```python
from build123d import *

# Parameters (mm, degrees)
SKETCH_1_W               = 65
SKETCH_1_H               = 25
EXTRUDE_1_DEPTH          = 20
EXTRUDE_2_DEPTH          = 65
SKETCH_3_W               = 50
SKETCH_3_H               = 20
CUT_EXTRUDE_1_DEPTH      = 15
CUT_EXTRUDE_2_DEPTH      = 50.33938589
CUT_EXTRUDE_2_DEPTH_BACK = 50.33938589
SKETCH_4_R               = 1.6
CUT_EXTRUDE_START        = -7
SKETCH_5_R               = 2.9
CUT_EXTRUDE_3_DEPTH      = 9
CUT_EXTRUDE_4_DEPTH      = 51.124844139
CUT_EXTRUDE_4_DEPTH_BACK = 51.124844139
SKETCH_6_R               = 1.6
FILLET_1_R               = 1


with BuildPart() as part:
    # 草图1 → 凸台-拉伸1 (new body)
    with BuildSketch(Plane(origin=(0, 0, 0), x_dir=(1, 0, 0), z_dir=(0, 1, 0))):
        Rectangle(SKETCH_1_W, SKETCH_1_H)
    extrude(amount=EXTRUDE_1_DEPTH)

    # 草图2 → 凸台-拉伸2 (add)
    with BuildSketch(Plane(origin=(32.5, 0, 0), x_dir=(0, 0, -1), z_dir=(1, 0, 0))):
        Polygon((-12.5, 0), (-32.5, 20), (-12.5, 20), align=None)
    extrude(amount=-EXTRUDE_2_DEPTH)

    # 草图3 → 切除-拉伸1 (cut)
    with BuildSketch(Plane.XZ):
        with Locations((0, -2.5)):
            Rectangle(SKETCH_3_W, SKETCH_3_H)
    extrude(amount=-CUT_EXTRUDE_1_DEPTH, mode=Mode.SUBTRACT)

    # 草图4 → 切除-拉伸2 (cut, two sides: drawn at the far end of the back side and taken through both)
    with BuildSketch(Plane(origin=(0, -6.25, 6.25), x_dir=(1, 0, 0), z_dir=(0, -0.7071067811865489, 0.7071067811865462)).offset(-CUT_EXTRUDE_2_DEPTH_BACK)):
        with Locations(Location((-22.5, 22.980970389, 0), (0, 0, 270))):
            Circle(SKETCH_4_R)
        with Locations(Location((22.5, 22.980970389, 0), (0, 0, 270))):
            Circle(SKETCH_4_R)
    extrude(amount=CUT_EXTRUDE_2_DEPTH + CUT_EXTRUDE_2_DEPTH_BACK, mode=Mode.SUBTRACT)

    # 草图5 → 切除-拉伸3 (cut)
    with BuildSketch(Plane(origin=(0, -6.25, 6.25), x_dir=(1, 0, 0), z_dir=(0, -0.7071067811865489, 0.7071067811865462)).offset(CUT_EXTRUDE_START)):
        with Locations(Location((-22.5, 22.980970389, 0), (0, 0, 270))):
            Circle(SKETCH_5_R)
        with Locations(Location((22.5, 22.980970389, 0), (0, 0, 320.160225214))):
            Circle(SKETCH_5_R)
    extrude(amount=-CUT_EXTRUDE_3_DEPTH, mode=Mode.SUBTRACT)

    # 草图6 → 切除-拉伸4 (cut, two sides: drawn at the far end of the back side and taken through both)
    with BuildSketch(Plane.XZ.offset(-CUT_EXTRUDE_4_DEPTH_BACK)):
        with Locations(Location((-28.75, 0, 0), (0, 0, 270))):
            Circle(SKETCH_6_R)
        with Locations(Location((28.75, 0, 0), (0, 0, 270))):
            Circle(SKETCH_6_R)
    extrude(amount=CUT_EXTRUDE_4_DEPTH + CUT_EXTRUDE_4_DEPTH_BACK, mode=Mode.SUBTRACT)

    # 圆角1
    fillet_1_edges = [part.edges().sort_by_distance(p)[0] for p in [
        (0, 20, 32.5),
    ]]
    fillet(fillet_1_edges, radius=FILLET_1_R)


solid = part.part
```
For this review, take the finished solid that the model builds, in its own axes (mm). A direction names the side the tool comes from. Coordinates: 2 decimals unless noted, no trailing zeros. Loops run counter-clockwise (first coordinate to the right, second up) from the corner with the lowest first, then second, coordinate; pieces in that order, holes last.
1. For faces 1 (the flat face through (0, 17, -12.5)), 2 (the flat face through (25, 7, -3)), 3 (the flat face through (-23.75, 14.07, 16.67)), list the 3-axis set-ups (+Z, -Z, +X, -X, +Y, -Y) from which the entire face can be reached by the end or side of a thin tool; tool diameter is ignored.
2. Mouldability with a two-part tool opening along Y and no side actions: class faces 4 (the cylindrical face through (30.336, 10.14, 0.208)), 5 (the flat face through (0, 20, 9)), 6 (the cylindrical face through (21.879, 15.377, 13.117)), 7 (the flat face through (0.5, 9, 21.5)) as +Y half, -Y half, draft (parallel to the pull), parting line (faces both ways), or undercut.
3. Add section D-D, the plane x = -5.5. Give the boundary of the cut face in (y, z).
4. For line 1 (X direction, y = 8.25, z = 0); line 2 (X direction, y = 1, z = -3); line 3 (Y direction, x = 16.5, z = -7.5), list the stretches that pass through material, from the lowest coordinate up.
5. Add section B-B, the plane y = 6.5. Give the boundary of the cut face in (x, z).
6. Insertion check: P1, Ø10, axis at x = 1, z = 0, coming from the -Y side; P2, Ø8, axis at x = 10.5, y = 2.5, coming from the -Z side; P3, Ø1.9, axis at x = 28.75, z = 0, coming from the +Y side; P4, Ø6, axis at x = 19.5, z = 21, coming from the -Y side. Each pin has a flat end and moves straight along its axis. Give the tip position at first contact, or say it passes through.
7. Add section A-A, the plane z = 0. Give the boundary of the cut face in (x, y).
8. Add section C-C, the plane x = 28.75. Give the boundary of the cut face in (y, z), then the cut area to 3 significant figures.
Result:
1. face 1: -Z, +X, -X, +Y, -Y
1. face 2: -Z, -Y
1. face 3: none
2. face 4: draft
2. face 5: +Y half
2. face 6: undercut
2. face 7: -Y half
3. outline: (0, 7.5) - (15, 7.5) - (15, -12.5) - (20, -12.5) - (20, 30.09) arc R1 ccw to (18.29, 30.79) - (0, 12.5) - close
4. line 1: x = -32.5 to -30.35, -27.15 to -25, 25 to 27.15, 30.35 to 32.5
4. line 2: x = -32.5 to -25, 25 to 32.5
4. line 3: y = 15 to 20
5. outline: (-32.5, -12.5) - (-25, -12.5) - (-25, 7.5) - (25, 7.5) - (25, -12.5) - (32.5, -12.5) - (32.5, 19) - (-32.5, 19) - close; hole circle Ø3.2 at (-28.75, 0); hole circle Ø3.2 at (28.75, 0)
6. P1: stops at y = 15
6. P2: stops at z = 7.5
6. P3: passes through
6. P4: stops at y = 5.5
7. outline: (-32.5, 0) - (-30.35, 0) - (-30.35, 20) - (-32.5, 20) - close; (-27.15, 0) - (-25, 0) - (-25, 15) - (25, 15) - (25, 0) - (27.15, 0) - (27.15, 20) - (-27.15, 20) - close; (30.35, 0) - (32.5, 0) - (32.5, 20) - (30.35, 20) - close
8. outline: (0, -12.5) - (20, -12.5) - (20, -1.6) - (0, -1.6) - close; (0, 1.6) - (20, 1.6) - (20, 30.09) arc R1 ccw to (18.29, 30.79) - (0, 12.5) - close
8. area: 635 mm2
